Could you check a few things on this drawing? It's one solid part, dimensions in mm from its lowest x, y, z. Round coordinates to 2 decimals unless told otherwise and drop trailing zeros. Write each loop counter-clockwise with the first axis right and the second up, starting at its lowest first coordinate (ties: lowest second). Pieces come first, ordered by that corner, then holes. Notation, with made-up numbers: (18.25, 4) -> (35.25, 4) arc R31 ccw to (35.25, 37) -> close; hole circle Ø8 at (-16, 12). An arc over 180 degrees is marked (long way). Answer in a Markdown table with one row per item.
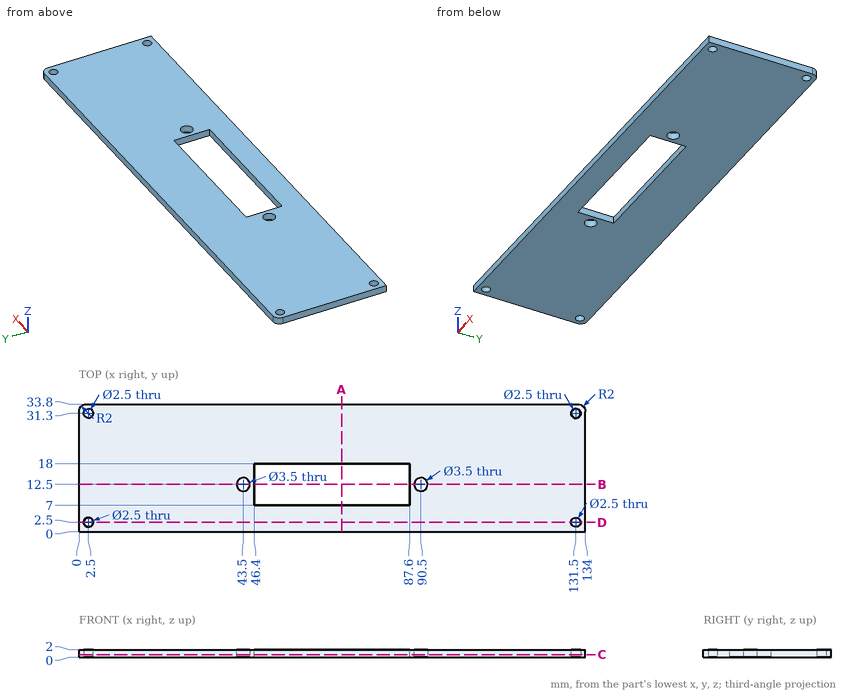
1) Imagine slicing it at A-A, the plane x = 69.5. Please give me the cut outline in (y, z).
Findings:
| item | result |
|---|---|
| outline | (0, 0) -> (7, 0) -> (7, 2) -> (0, 2) -> close; (18, 0) -> (33.8, 0) -> (33.8, 2) -> (18, 2) -> close |
2) Please list where these lines run through material, in increasing order: line 1 (Y direction, x = 131.5, z = 0.7); line 2 (X direction, y = 31.3, z = 0.6); line 3 (X direction, y = 7.5, z = 1.15).
Findings:
| item | result |
|---|---|
| line 1 | y = 0 to 1.25, 3.75 to 30.05, 32.55 to 33.8 |
| line 2 | x = 0 to 1.25, 3.75 to 130.25, 132.75 to 134 |
| line 3 | x = 0 to 46.4, 87.6 to 134 |
3) For pin 1 (3 mm diameter, centred on x = 131.5, y = 2.5, fed in from -Z), with a flat end and sliding along its axis, tell me the tip position at first contact or that it passes through.
Findings:
| item | result |
|---|---|
| pin 1 | stops at z = 0 |
4) Imagine slicing it at B-B, the plane y = 12.5. Please give me the cut outline in (x, z).
Findings:
| item | result |
|---|---|
| outline | (0, 0) -> (41.75, 0) -> (41.75, 2) -> (0, 2) -> close; (45.25, 0) -> (46.4, 0) -> (46.4, 2) -> (45.25, 2) -> close; (87.6, 0) -> (88.75, 0) -> (88.75, 2) -> (87.6, 2) -> close; (92.25, 0) -> (134, 0) -> (134, 2) -> (92.25, 2) -> close |
5) Imagine slicing it at D-D, the plane y = 2.5. Please give me the cut outline in (x, z), plus the area to 3 significant figures.
Findings:
| item | result |
|---|---|
| outline | (0, 0) -> (1.25, 0) -> (1.25, 2) -> (0, 2) -> close; (3.75, 0) -> (130.25, 0) -> (130.25, 2) -> (3.75, 2) -> close; (132.75, 0) -> (134, 0) -> (134, 2) -> (132.75, 2) -> close |
| area | 258 mm^2 |
6) Imagine slicing it at C-C, the plane z = 0.7. Please give me the cut outline in (x, y).
Findings:
| item | result |
|---|---|
| outline | (0, 0) -> (134, 0) -> (134, 31.8) arc R2 ccw to (132, 33.8) -> (2, 33.8) arc R2 ccw to (0, 31.8) -> close; hole circle Ø2.5 at (2.5, 2.5); hole circle Ø2.5 at (2.5, 31.3); hole circle Ø3.5 at (43.5, 12.5); hole (46.4, 7) -> (87.6, 7) -> (87.6, 18) -> (46.4, 18) -> close; hole circle Ø3.5 at (90.5, 12.5); hole circle Ø2.5 at (131.5, 2.5); hole circle Ø2.5 at (131.5, 31.3) |
